from build123d import *

# Parameters (mm, degrees)
BOSS_EXTRUDE1_DEPTH = 7
SKETCH5_R           = 2
CUT_EXTRUDE2_DEPTH  = 8
BOSS_EXTRUDE2_DEPTH = 40
CUT_EXTRUDE3_DEPTH  = 48
BOSS_EXTRUDE3_DEPTH = 7
BOSS_EXTRUDE4_DEPTH = 7
FILLET1_R           = 5
SKETCH10_W          = 50
SKETCH10_H          = 40
CUT_EXTRUDE4_DEPTH  = 117.99261314
FILLET2_R           = 10
SKETCH11_R          = 2
CUT_EXTRUDE5_DEPTH  = 8


with BuildPart() as part:
    # Sketch4 → Boss-Extrude1 (new body)
    with BuildSketch(Plane.XY):
        with BuildLine():
            Line((-13.856406461, 8), (-35.606406461, -29.672105065))
            Line((-35.606406461, -29.672105065), (-22.616025404, -37.172105065))
            Line((-22.616025404, -37.172105065), (-35.116025404, -58.822740159))
            Line((-35.116025404, -58.822740159), (-48.106406461, -51.322740159))
            Line((-48.106406461, -51.322740159), (-70, 60))
            Line((-70, 60), (70, 60))
            Line((70, 60), (48.106406461, -51.322740159))
            Line((48.106406461, -51.322740159), (35.116025404, -58.822740159))
            Line((35.116025404, -58.822740159), (22.616025404, -37.172105065))
            Line((22.616025404, -37.172105065), (35.606406461, -29.672105065))
            Line((35.606406461, -29.672105065), (13.856406461, 8))
            ThreePointArc((13.856406461, 8), (0, 16), (-13.856406461, 8))
        make_face()
    extrude(amount=BOSS_EXTRUDE1_DEPTH)

    # Sketch5 → Cut-Extrude2 (cut, through all)
    with BuildSketch(Plane.XY):
        with Locations((-39.11, -50.743315159)):
            Circle(SKETCH5_R)
        with Locations((-31.61, -37.752934102)):
            Circle(SKETCH5_R)
        with Locations((39.11, -50.743315159)):
            Circle(SKETCH5_R)
        with Locations((31.61, -37.752934102)):
            Circle(SKETCH5_R)
    extrude(amount=CUT_EXTRUDE2_DEPTH, mode=Mode.SUBTRACT)

    # Sketch6 → Boss-Extrude2 (add)
    with BuildSketch(Plane.XY.offset(7)):
        Polygon((-68.623325705, 53), (68.623325705, 53), (70, 60), (-70, 60), align=None)
    extrude(amount=BOSS_EXTRUDE2_DEPTH)

    # Sketch7 → Cut-Extrude3 (cut, through all)
    with BuildSketch(Plane.XY.offset(47)):
        Polygon((-68.623325705, 53), (-68.623325705, 60), (-70, 60), align=None)
        Polygon((68.623325705, 53), (68.623325705, 60), (70, 60), align=None)
    extrude(amount=-CUT_EXTRUDE3_DEPTH, mode=Mode.SUBTRACT)

    # Sketch8 → Boss-Extrude3 (add)
    with BuildSketch(Plane.ZY.offset(35)):
        Polygon((7, 13), (47, 53), (7, 53), align=None)
    extrude(amount=BOSS_EXTRUDE3_DEPTH)

    # Sketch9 → Boss-Extrude4 (add)
    with BuildSketch(Plane(origin=(35, 0, 0), x_dir=(0, 0, -1), z_dir=(1, 0, 0))):
        Polygon((-7, 13), (-47, 53), (-7, 53), align=None)
    extrude(amount=BOSS_EXTRUDE4_DEPTH)

    # Fillet1
    fillet1_edges = [part.edges().sort_by_distance(p)[0] for p in [
        (-35.606406461, -29.672105065, 3.5),
        (-22.616025404, -37.172105065, 3.5),
        (-35.116025404, -58.822740159, 3.5),
        (-48.106406461, -51.322740159, 3.5),
        (48.106406461, -51.322740159, 3.5),
        (35.116025404, -58.822740159, 3.5),
        (22.616025404, -37.172105065, 3.5),
        (35.606406461, -29.672105065, 3.5),
    ]]
    fillet(fillet1_edges, radius=FILLET1_R)

    # Sketch10 → Cut-Extrude4 (cut, through all)
    with BuildSketch(Plane(origin=(0, 60, 0), x_dir=(1, 0, 0), z_dir=(0, 1, 0))):
        with Locations((0, -27)):
            Rectangle(SKETCH10_W, SKETCH10_H)
    extrude(amount=-CUT_EXTRUDE4_DEPTH, mode=Mode.SUBTRACT)

    # Fillet2
    fillet2_edges = [part.edges().sort_by_distance(p)[0] for p in [
        (25, 56.5, 47),
        (-25, 56.5, 47),
        (-68.623325705, 56.5, 47),
        (68.623325705, 56.5, 47),
    ]]
    fillet(fillet2_edges, radius=FILLET2_R)

    # Sketch11 → Cut-Extrude5 (cut, through all)
    with BuildSketch(Plane.XZ.offset(-53)):
        with Locations((-59.748883804, 33.666666667)):
            Circle(SKETCH11_R)
        with Locations((-50.874441902, 33.666666667)):
            Circle(SKETCH11_R)
        with Locations((-59.748883804, 20.333333333)):
            Circle(SKETCH11_R)
        with Locations((-50.874441902, 20.333333333)):
            Circle(SKETCH11_R)
        with Locations((50.874441902, 20.333333333)):
            Circle(SKETCH11_R)
        with Locations((59.748883804, 20.333333333)):
            Circle(SKETCH11_R)
        with Locations((50.874441902, 33.666666667)):
            Circle(SKETCH11_R)
        with Locations((59.748883804, 33.666666667)):
            Circle(SKETCH11_R)
    extrude(amount=-CUT_EXTRUDE5_DEPTH, mode=Mode.SUBTRACT)


solid = part.part
Part model, mm, in its own coordinate system. A direction names the side the tool comes from. Round coordinates to 2 decimals unless told otherwise and drop trailing zeros. Write each loop counter-clockwise with the first axis right and the second up, starting at its lowest first coordinate (ties: lowest second). Pieces come first, ordered by that corner, then holes. Notation, with made-up numbers: M -9.75,-23 L 21.25,-23 A19 cw 21.25,-9 Z; hole C 29.25,31 d10. An arc over 180 degrees is marked long. Return JSON: item names as keys, results as strings. Group by question number.
(1) Saw through at A-A on z = 13. Write the cut outline in (x, y), then the cut area to 3 significant figures.
(2) Saw through at B-B on y = -19. Write the cut outline in (x, z).
(3) Which spindle directions (+Z, -Z, +X, -X, +Y, -Y) get a long thin tool onto all of the face, cutting with end or side? Do faces 4 (the face through (30, 53, 27)), 5 (the face through (-29.142, -33.405, 3.451)), 6 (the face through (28.01, 56.45, 44.15)). Say none if no direction does.
(4) Saw through at C-C on z = 5. Write the cut outline in (x, y), then the cut area to 3 significant figures.
(5) Saw through at D-D on x = 0. Write the cut outline in (y, z).
(6) Drill centre lines: probe 1 along X at (y, z) = (35, 23.5); probe 2 along Y at (x, z) = (31, 3); probe 3 along Z at (x, y) = (-48, -2). Where is each one in solid material? Low to high.
(7) Pin check, flat tips, straight feed: pin 1 Ø5 at (x, y) = (-31.61, -37.75) entering from +Z; pin 2 Ø2.5 at (x, z) = (50.87, 33.67) entering from +Y; pin 3 Ø21.5 at (x, z) = (-58, 22) entering from -Y; pin 4 Ø20 at (y, z) = (41.5, 20) entering from -X. Stop position of each tip, or through.
(8) Two-plate mould, pull along X, no slides. Class faces 1 (the face through (68.623, 56, 19)), 2 (the face through (-42, 38, 22)), 3 (the face through (-25, 57, 22)): +X half, -X half, draft (parallel to the pull), parting line (faces both ways), or undercut.
Returned:
{
 "1": {"outline": "M -68.62,53 L -42,53 L -42,19 L -35,19 L -35,53 L -25,53 L -25,60 L -68.62,60 Z; M 25,53 L 35,53 L 35,19 L 42,19 L 42,53 L 68.62,53 L 68.62,60 L 25,60 Z", "area": "1,090 mm²"},
 "2": {"outline": "M -54.46,0 L -29.44,0 L -29.44,7 L -54.46,7 Z; M 29.44,0 L 54.46,0 L 54.46,7 L 29.44,7 Z"},
 "3": {"face 4": "+Z, -Y", "face 5": "+Z, -Z", "face 6": "+Z, +Y, -Y"},
 "4": {"outline": "M -68.62,53 L -48.54,-49.09 A5 ccw -46.14,-52.46 L -39.45,-56.32 A5 ccw -32.62,-54.49 L -25.12,-41.5 A5 ccw -26.95,-34.67 L -31.28,-32.17 A5 cw -33.11,-25.34 L -13.86,8 A16 cw 13.86,8 L 33.11,-25.34 A5 cw 31.28,-32.17 L 26.95,-34.67 A5 ccw 25.12,-41.5 L 32.62,-54.49 A5 ccw 39.45,-56.32 L 46.14,-52.46 A5 ccw 48.54,-49.09 L 68.62,53 L 68.62,60 L -68.62,60 Z; hole C -39.11,-50.74 d4; hole C -31.61,-37.75 d4; hole C 31.61,-37.75 d4; hole C 39.11,-50.74 d4", "area": "9,990 mm²"},
 "5": {"outline": "M 16,0 L 60,0 L 60,7 L 16,7 Z"},
 "6": {"probe 1": "-42 to -35, 35 to 42", "probe 2": "-51.69 to -39.66, -35.85 to -32.33, -21.69 to 60", "probe 3": "0 to 7"},
 "7": {"pin 1": "z = 7", "pin 2": "through", "pin 3": "y = 53", "pin 4": "x = -42"},
 "8": {"face 1": "+X half", "face 2": "-X half", "face 3": "undercut"}
}
